Here's how the part is built. I have some questions about the finished solid (model axes, mm). Face numbers are marked on the shaded views. A direction names the side the tool comes from. Coordinates: 2 decimals unless noted, no trailing zeros. Loops run counter-clockwise (first coordinate to the right, second up) from the corner with the lowest first, then second, coordinate; pieces in that order, holes last. Notation, with made-up numbers: M 49.5,73 L 64.5,73 A24 ccw 64.5,90 Z; hole C 8,-24 d11. An arc over 180 degrees is marked long. Use CSV: the item, a comma, the result in double quotes. Start each with the question number.
Q1. If we section it at D-D (x = 30.5): Please give me the cut outline in (y, z), and give its area (3 significant figures).
Q2. For pin 1 Ø7.5 at (x, y) = (63, -11) entering from +Z (3 decimals); pin 2 Ø12 at (y, z) = (-10, 55.5) entering from +X; pin 3 Ø2 at (y, z) = (-14, 18.5) entering from +X, each with a flat end and sliding along its axis, tell me the tip position at first contact or that it passes through.
Q3. If we section it at A-A (z = 36): Please give me the cut outline in (x, y), and give its area (3 significant figures).
Q4. If we section it at B-B (y = -18.25): Please give me the cut outline in (x, z) (1 decimal).
Q5. Please list where these lines run through material, in increasing order: probe 1 along Z at (x, y) = (-59.5, -23) (3 decimals); probe 2 along X at (y, z) = (-23.25, 72.5); probe 3 along X at (y, z) = (-8.25, 71). Write a range as [from, to].
Q6. If we mould it in two halves opening along X, with no side actions, what happens to the marked faces 1, 2 and 3? For each: +X half, -X half, draft (parallel to the pull), parting line (faces both ways), or undercut.
Q7. If we section it at C-C (x = 59): Please give me the cut outline in (y, z) (3 decimals), and give its area (3 significant figures).
Q8. Which directions (+Z, -Z, +X, -X, +Y, -Y) give clear straight access to the entire face, cutting with the end or side of a thin tool? Please do the marked faces 4, 5, 6 and 7.
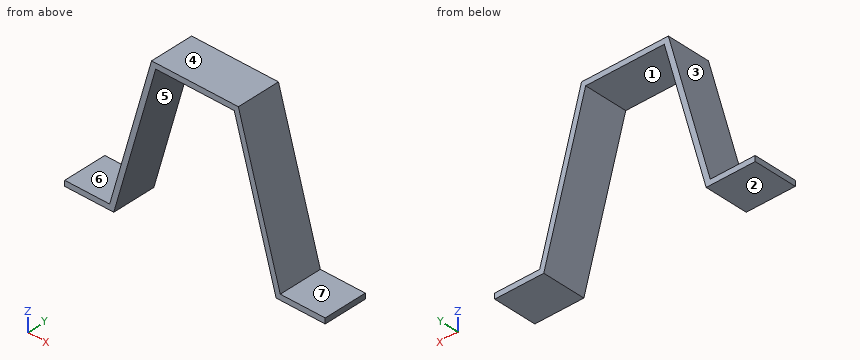
from build123d import *

# Parameters (mm, degrees)
F1_DEPTH = 25.4
F2_W     = 28.575
F2_H     = 25.4
F3_DEPTH = 3.175


with BuildPart() as f1:
    # F0 (on Front) → F1 (new body)
    with BuildSketch(Plane.XZ):
        Polygon((-22.998106, 86.6775), (0, 86.6775), (0, 89.8525), (-25.4, 89.8525), (-50.8, 0), (-47.500579, 0), align=None)
        Polygon((22.998106, 86.6775), (47.500579, 0), (50.8, 0), (25.4, 89.8525), (0, 89.8525), (0, 86.6775), align=None)
    extrude(amount=F1_DEPTH)

    # F2 (on Top) → F3 (join)
    with BuildSketch(Plane.XY):
        with Locations((-61.9125, -12.7)):
            Rectangle(F2_W, F2_H)
        with Locations((61.9125, -12.7)):
            Rectangle(F2_W, F2_H)
    extrude(amount=F3_DEPTH)


solid = f1.part
Results below:
1,outline,"M -25.4,60.14 L 0,60.14 L 0,71.81 L -25.4,71.81 Z"
1,area,"296 mm^2"
2,pin 1,"z = 3.175"
2,pin 2,"x = 36.81"
2,pin 3,"x = 45.85"
3,outline,"M -40.62,-25.4 L -37.32,-25.4 L -37.32,0 L -40.62,0 Z; M 37.32,-25.4 L 40.62,-25.4 L 40.62,0 L 37.32,0 Z"
3,area,"168 mm^2"
4,outline,"M -76.2,0 L -47.5,0 L -23,86.7 L 23,86.7 L 47.5,0 L 76.2,0 L 76.2,3.2 L 49.9,3.2 L 25.4,89.9 L -25.4,89.9 L -49.9,3.2 L -76.2,3.2 Z"
5,probe 1,"[0, 3.175]"
5,probe 2,"[-30.31, -27.01], [27.01, 30.31]"
5,probe 3,"[-30.73, -27.43], [27.43, 30.73]"
6,face 1,"undercut"
6,face 2,"draft"
6,face 3,"-X half"
7,outline,"M -25.4,0 L 0,0 L 0,3.175 L -25.4,3.175 Z"
7,area,"80.6 mm^2"
8,face 4,"+Z, +X, -X, +Y, -Y"
8,face 5,"-Z, +Y, -Y"
8,face 6,"+Z, -X, +Y, -Y"
8,face 7,"+Z, +X, +Y, -Y"
